Geometry check sheet. Reference: the model listing, model coordinates, mm. Face numbers are marked on the shaded views. A direction names the side the tool comes from. Coordinates: 2 decimals unless noted, no trailing zeros. Loops run counter-clockwise (first coordinate to the right, second up) from the corner with the lowest first, then second, coordinate; pieces in that order, holes last. Notation, with made-up numbers: (8.25, 71) - (41.25, 71) arc R20 ccw to (41.25, 75) - close; hole circle Ø7 at (6.25, 20). An arc over 180 degrees is marked (long way). Write item = value, one per line. Start each with the question number.
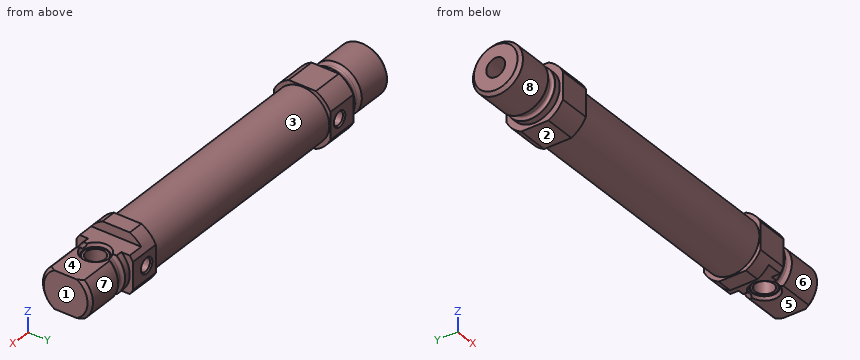
from build123d import *

# Parameters (mm, degrees)
BOSS_EXTRUDE1_DEPTH     = 10
SKETCH3_W               = 76
SKETCH3_H               = 8.65
SKETCH4_W               = 18
SKETCH4_H               = 18
BOSS_EXTRUDE2_DEPTH     = 10
SKETCH5_W               = 10
SKETCH5_H               = 10
CUT_EXTRUDE1_DEPTH      = 10
CUT_EXTRUDE1_DEPTH_BACK = 10
HOLE1_D                 = 4.134
HOLE1_DEPTH             = 9
HOLE1_CSINK_D           = 5
HOLE1_CSINK_ANGLE       = 90
HOLE2_D                 = 4.134
HOLE2_DEPTH             = 11
HOLE2_CSINK_D           = 5
HOLE2_CSINK_ANGLE       = 90
HOLE2_TIP               = 1.193383006


with BuildPart() as part:
    # Sketch1 → Revolve1 (revolve)
    with BuildSketch(Plane.XY):
        with BuildLine():
            Line((0, 0), (0, 7))
            Line((0, 7), (1, 8))
            Line((1, 8), (11.95, 8))
            Line((11.95, 8), (12.865685425, 7.084314575))
            ThreePointArc((12.865685425, 7.084314575), (13.125224104, 6.910896374), (13.43137085, 6.85))
            Line((13.43137085, 6.85), (14.2, 6.85))
            ThreePointArc((14.2, 6.85), (14.765685425, 7.084314575), (15, 7.65))
            Line((15, 7.65), (15, 8))
            Line((15, 8), (17, 8))
            Line((17, 8), (17, 0))
            Line((17, 0), (0, 0))
        make_face()
    revolve(axis=Axis((17, 0, 0), (-1, 0, 0)))

    # Sketch2 → Boss-Extrude1 (add)
    with BuildSketch(Plane(origin=(17, 0, 0), x_dir=(0, 0, -1), z_dir=(1, 0, 0))):
        with BuildLine():
            Line((-4.358898944, -9), (4.358898944, -9))
            ThreePointArc((4.358898944, -9), (7.071067812, -7.071067812), (9, -4.358898944))
            Line((9, -4.358898944), (9, 4.358898944))
            ThreePointArc((9, 4.358898944), (7.071067812, 7.071067812), (4.358898944, 9))
            Line((4.358898944, 9), (-4.358898944, 9))
            ThreePointArc((-4.358898944, 9), (-7.071067812, 7.071067812), (-9, 4.358898944))
            Line((-9, 4.358898944), (-9, -4.358898944))
            ThreePointArc((-9, -4.358898944), (-7.071067812, -7.071067812), (-4.358898944, -9))
        make_face()
    extrude(amount=BOSS_EXTRUDE1_DEPTH)

    # Sketch3 → Revolve2 (revolve)
    with BuildSketch(Plane.XY):
        with Locations((65, 4.325)):
            Rectangle(SKETCH3_W, SKETCH3_H)
    revolve(axis=Axis((103, 0, 0), (-1, 0, 0)))

    # Sketch4 → Boss-Extrude2 (add)
    with BuildSketch(Plane(origin=(103, 0, 0), x_dir=(0, 0, -1), z_dir=(1, 0, 0))):
        Rectangle(SKETCH4_W, SKETCH4_H)
    extrude(amount=BOSS_EXTRUDE2_DEPTH)

    # Sketch5 → Cut-Revolve1 (revolve, cut)
    with BuildSketch(Plane.XY):
        with Locations((108, 15)):
            Rectangle(SKETCH5_W, SKETCH5_H)
    revolve(axis=Axis((113, 0, 0), (-1, 0, 0)), mode=Mode.SUBTRACT)

    # Sketch6 → Revolve3 (revolve)
    with BuildSketch(Plane.XY):
        with BuildLine():
            Line((113, 0), (113, 8))
            Line((113, 8), (115, 8))
            Line((115, 8), (115, 7.65))
            ThreePointArc((115, 7.65), (115.234314575, 7.084314575), (115.8, 6.85))
            Line((115.8, 6.85), (116.56862915, 6.85))
            ThreePointArc((116.56862915, 6.85), (116.874775896, 6.910896374), (117.134314575, 7.084314575))
            Line((117.134314575, 7.084314575), (118.05, 8))
            Line((118.05, 8), (129, 8))
            Line((129, 8), (130, 7))
            Line((130, 7), (130, 0))
            Line((130, 0), (113, 0))
        make_face()
    revolve(axis=Axis((130, 0, 0), (-1, 0, 0)))

    # Sketch7 → Cut-Extrude1 (cut, two sides)
    with BuildSketch(Plane(origin=(0, 0, 0), x_dir=(1, 0, 0), z_dir=(0, 1, 0))) as cut_extrude1_sk:
        Polygon((108, 18), (108, 6), (130, 6), (130, -6), (108, -6), (108, -18), (142, -18), (142, 18), align=None)
    extrude(amount=CUT_EXTRUDE1_DEPTH, mode=Mode.SUBTRACT)
    extrude(cut_extrude1_sk.sketch, amount=-CUT_EXTRUDE1_DEPTH_BACK, mode=Mode.SUBTRACT)

    # Sketch8 → Cut-Revolve2 (revolve, cut)
    with BuildSketch(Plane(origin=(117, 0, 0), x_dir=(0, 0, -1), z_dir=(1, 0, 0))):
        Polygon((-6.2, 0), (-6.2, 4.692820323), (-5, 4), (-4.5, 4), (-5, 3.711324865), (-5, 3), (5, 3), (5, 3.711324865), (4.5, 4), (5, 4), (6.2, 4.692820323), (6.2, 0), align=None)
    revolve(axis=Axis((117, 0, -5), (0, 0, 1)), mode=Mode.SUBTRACT)

    # Hole1
    with Locations(Plane(origin=(0, 9, 0), x_dir=(1, 0, 0), z_dir=(0, 1, 0))):
        with Locations((23, 0)):
            CounterSinkHole(HOLE1_D / 2, HOLE1_CSINK_D / 2, depth=HOLE1_DEPTH, counter_sink_angle=HOLE1_CSINK_ANGLE)

    # Hole2
    with Locations(Plane(origin=(0, 9, 0), x_dir=(1, 0, 0), z_dir=(0, 1, 0))):
        with Locations((107, 0)):
            CounterSinkHole(HOLE2_D / 2, HOLE2_CSINK_D / 2, depth=HOLE2_DEPTH, counter_sink_angle=HOLE2_CSINK_ANGLE)
            with Locations((0, 0, -(HOLE2_DEPTH + HOLE2_TIP / 2))):  # 120° drill point
                Cone(0, HOLE2_D / 2, HOLE2_TIP, mode=Mode.SUBTRACT)

    # Sketch13 → Cut-Revolve3 (revolve, cut)
    with BuildSketch(Plane.XY):
        Polygon((-5, 0), (-5, 3), (41.2, 3), (41.2, 8), (85.2, 8), (85.2, 0), align=None)
    revolve(axis=Axis((85.2, 0, 0), (-1, 0, 0)), mode=Mode.SUBTRACT)


solid = part.part
(1) Sectioned sample at C-C on x = 9. Enter the section's corners in (y, z), plus the area to 3 significant figures.
(2) Sectioned sample at A-A on y = 0. Count the separate pieces of the cut face and the enclosed holes in it, plus the area to 3 significant figures.
(3) Draft check along X on the marked faces 1, 2 and 3. Enter one of: pulls with the +X half, pulls with the -X half, needs draft (parallel to the pull), parting line crosses it, or undercut.
(4) Scan lines: line 1 (Z direction, x = 75, y = 0); line 2 (Y direction, x = 29, z = 0); line 3 (Z direction, x = 8, y = -0.25). Record each from-to range of solid material in increasing order.
(5) Depth check by flat-ended pin: pin 1 (5.5 mm diameter, centred on x = 111, y = 0, fed in from -Z); pin 2 (2 mm diameter, centred on x = 113.5, y = -0.5, fed in from +Z); pin 3 (5 mm diameter, centred on x = 36, z = -2, fed in from -Y). Enter the tip coordinate at first touch or a pass-through.
(6) Tool access check on the marked faces 4, 5, 6, 7 and 8. Record the directions out of +Z, -Z, +X, -X, +Y, -Y that give a thin tool (end or side, any length) a straight path to the whole face; none if there is none.
(7) Sectioned sample at B-B on x = 23. Enter the section's corners in (y, z).
Working result:
q1.outline = circle Ø16 at (0, 0); hole circle Ø6 at (0, 0)
q1.area = 173 mm2
q2.separate_pieces = 2
q2.enclosed_holes = 1
q2.area = 1,070 mm2
q3.face_1 = pulls with the +X half
q3.face_2 = needs draft
q3.face_3 = undercut
q4.line_1 = -8.65 to -8, 8 to 8.65
q4.line_2 = -8.65 to -3, 3 to 8.65
q4.line_3 = -8 to -2.99, 2.99 to 8
q5.pin_1 = -6
q5.pin_2 = 5.93
q5.pin_3 = -8.65
q6.face_4 = +Z, +X, +Y, -Y
q6.face_5 = -Z, +X, +Y, -Y
q6.face_6 = +X, -Y
q6.face_7 = +X, +Y
q6.face_8 = -X
q7.outline = (-9, -4.36) arc R10 ccw to (-4.36, -9) - (4.36, -9) arc R10 ccw to (9, -4.36) - (9, -2.5) - (8.57, -2.07) - (2.17, -2.07) arc R3 cw (long way) to (2.17, 2.07) - (8.57, 2.07) - (9, 2.5) - (9, 4.36) arc R10 ccw to (4.36, 9) - (-4.36, 9) arc R10 ccw to (-9, 4.36) - close
